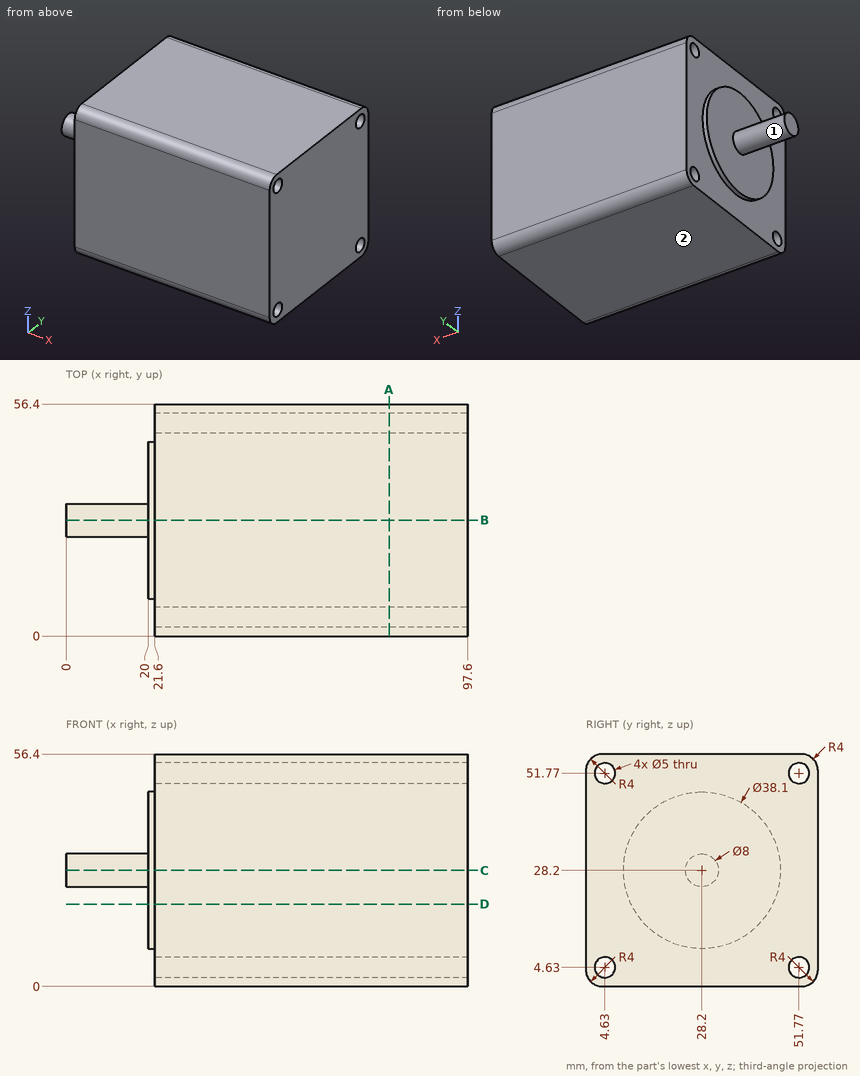
Part print with two shaded views. Sizes in mm from the minimum x, y, z corner. A direction names the side the tool comes from. Give positions to 0.01 mm unless a question says otherwise; leave off trailing zeros. Order: outer loops, then holes, each group sorted by start corner. A loop starts at its lowest first (then second) coordinate and runs counter-clockwise, first axis right, second up.
1) Wall check: probe 1 along Z at (x, y) = (62, 4.63); probe 2 along Y at (x, z) = (61, 4). Give the ranges that are in metal, low to high.
2) Saw through at A-A, the plane x = 78.5. Write the cut outline in (y, z).
3) Pin check, flat tips, straight feed: pin 1 (8 mm diameter, centred on y = 4.63, z = 4.63, fed in from +X); pin 2 (4 mm diameter, centred on y = 51.77, z = 4.63, fed in from +X); pin 3 (6 mm diameter, centred on y = 36, z = 21, fed in from -X). Stop position of each tip, or through.
4) Saw through at D-D, the plane z = 20. Write the cut outline in (x, y), then the cut area to 3 significant figures.
5) Saw through at B-B, the plane y = 28.2. Write the cut outline in (x, z), then the cut area to 3 significant figures.
6) 3-axis set-ups, long thin cutter, end or side, ignore diameter. For the marked faces 1 and 2: which of +Z, -Z, +X, -X, +Y, -Y reach the whole face in a straight line?
Computed:
1. probe 1: z = 0 to 2.13, 7.13 to 49.27, 54.27 to 56.4
1. probe 2: y = 0 to 2.21, 7.05 to 49.35, 54.19 to 56.4
2. outline: (0, 4) arc R4 ccw to (4, 0) - (52.4, 0) arc R4 ccw to (56.4, 4) - (56.4, 52.4) arc R4 ccw to (52.4, 56.4) - (4, 56.4) arc R4 ccw to (0, 52.4) - close; hole circle Ø5 at (4.63, 4.63); hole circle Ø5 at (4.63, 51.77); hole circle Ø5 at (51.77, 4.63); hole circle Ø5 at (51.77, 51.77)
3. pin 1: stops at x = 97.6
3. pin 2: passes through
3. pin 3: stops at x = 20
4. outline: (20, 11.01) - (21.6, 11.01) - (21.6, 0) - (97.6, 0) - (97.6, 56.4) - (21.6, 56.4) - (21.6, 45.39) - (20, 45.39) - close
4. area: 4,340 mm2
5. outline: (0, 24.2) - (20, 24.2) - (20, 9.15) - (21.6, 9.15) - (21.6, 0) - (97.6, 0) - (97.6, 56.4) - (21.6, 56.4) - (21.6, 47.25) - (20, 47.25) - (20, 32.2) - (0, 32.2) - close
5. area: 4,510 mm2
6. face 1: -X
6. face 2: -Z, +X, -X, +Y, -Y
